```python
from build123d import *

# Parameters (mm, degrees)
F1_DEPTH = 5
F0_W     = 3
F0_H     = 25
F2_DEPTH = 0.2
F3_DEPTH = 0.3
F4_DEPTH = 0.4
F5_DEPTH = 0.5
F6_DEPTH = 0.6


with BuildPart() as f1:
    # F0 (on Top) → F1 (new body)
    with BuildSketch(Plane.XY):
        Polygon((-7.5, -15), (7.5, -15), (7.5, -10), (4.5, -10), (1.5, -10), (-1.5, -10), (-4.5, -10), (-7.5, -10), align=None)
    extrude(amount=F1_DEPTH)

    # F0 (on Top) → F2 (join)
    with BuildSketch(Plane.XY):
        with Locations((-6, 2.5)):
            Rectangle(F0_W, F0_H)
    extrude(amount=F2_DEPTH)

    # F0 (on Top) → F3 (join)
    with BuildSketch(Plane.XY):
        with Locations((-3, 2.5)):
            Rectangle(F0_W, F0_H)
    extrude(amount=F3_DEPTH)

    # F0 (on Top) → F4 (join)
    with BuildSketch(Plane.XY):
        with Locations((0, 2.5)):
            Rectangle(F0_W, F0_H)
    extrude(amount=F4_DEPTH)

    # F0 (on Top) → F5 (join)
    with BuildSketch(Plane.XY):
        with Locations((3, 2.5)):
            Rectangle(F0_W, F0_H)
    extrude(amount=F5_DEPTH)

    # F0 (on Top) → F6 (join)
    with BuildSketch(Plane.XY):
        with Locations((6, 2.5)):
            Rectangle(F0_W, F0_H)
    extrude(amount=F6_DEPTH)


solid = f1.part
```
Input: part model. Units: mm. Frame: model coordinates. A direction names the side the tool comes from. Coordinates: 2 decimals unless noted, no trailing zeros. Write each loop counter-clockwise with the first axis right and the second up, starting at its lowest first coordinate (ties: lowest second). Pieces come first, ordered by that corner, then holes. Notation, with made-up numbers: (-18, -26.75) -> (34, -26.75) arc R17 cw to (34, -0.75) -> close; hole circle Ø5 at (77.25, -24.5). An arc over 180 degrees is marked (long way). Answer as a JSON object with one key per item and string values.
1. Section D-D on x = 4. Return the cut outline in (y, z), then the cut area to 3 significant figures.
Result set:
{"outline": "(-15, 0) -> (15, 0) -> (15, 0.5) -> (-10, 0.5) -> (-10, 5) -> (-15, 5) -> close", "area": "37.5 mm2"}
2. Material intervals for line 1 (Y direction, x = 2.75, z = 1.65); line 2 (Z direction, x = -5.5, y = -4); line 3 (Z direction, x = 4, y = 6.5), sorted ascending. Write a range as from..to.
Result set:
{"line 1": "y = -15..-10", "line 2": "z = 0..0.2", "line 3": "z = 0..0.5"}
3. Section A-A on x = 0.5. Return the cut outline in (y, z).
Result set:
{"outline": "(-15, 0) -> (15, 0) -> (15, 0.4) -> (-10, 0.4) -> (-10, 5) -> (-15, 5) -> close"}
4. Section C-C on z = 1.5. Return the cut outline in (x, y), then the cut area to 3 significant figures.
Result set:
{"outline": "(-7.5, -15) -> (7.5, -15) -> (7.5, -10) -> (-7.5, -10) -> close", "area": "75.0 mm2"}
5. Section B-B on y = 9. Return the cut outline in (x, z), then the cut area to 3 significant figures.
Result set:
{"outline": "(-7.5, 0) -> (7.5, 0) -> (7.5, 0.6) -> (4.5, 0.6) -> (4.5, 0.5) -> (1.5, 0.5) -> (1.5, 0.4) -> (-1.5, 0.4) -> (-1.5, 0.3) -> (-4.5, 0.3) -> (-4.5, 0.2) -> (-7.5, 0.2) -> close", "area": "6.00 mm2"}
6. First-contact query: P1, Ø0.9, axis at x = -6, y = 8, coming from the +Z side; P2, Ø4, axis at x = 5, y = -2, coming from the +Z side; P3, Ø0.9, axis at x = 0.5, y = 8, coming from the +Z side; P4, Ø4, axis at x = -2, y = 1.5, coming from the -Z side. Flat tips, straight axial feed; report the tip coordinate or a pass-through.
Result set:
{"P1": "stops at z = 0.2", "P2": "stops at z = 0.6", "P3": "stops at z = 0.4", "P4": "stops at z = 0"}
7. Access query for faces 1 (the face through (6, 3, 0.6)), 2 (the face through (0, -12, 5)), 3 (the face through (3, 3, 0.5)). Directions: +Z, -Z, +X, -X, +Y, -Y. A direction counts if a zero-diameter tool reaches every point of the face in a straight line with its end or side. Return the directions, or none.
Result set:
{"face 1": "+Z, +X, -X, +Y", "face 2": "+Z, +X, -X, +Y, -Y", "face 3": "+Z, -X, +Y"}
